Study the drawing (mm; zero at the part's minimum x, y, z) and answer. A direction names the side the tool comes from. Round coordinates to 2 decimals unless told otherwise and drop trailing zeros. Loops run counter-clockwise (first coordinate to the right, second up) from the corner with the lowest first, then second, coordinate; pieces in that order, holes last. Notation, with made-up numbers: M 14.25,57.25 L 50.25,57.25 A8 ccw 50.25,70.25 Z; hole C 35.5,-14.75 d3. An arc over 180 degrees is marked long. Put each result on its own line as item: value. Start each with the question number.
(1) Section B-B, the plane x = 2.25 is taken. Determine the outline of the cut face in (y, z), then the cut area to 4 significant figures.
(2) Determine the mould class of the marked faces 6, 7 and 8 for opening direction X: released by +X, released by -X, zero draft, split by the parting line, or undercut.
(3) Which of the six approach directions +Z, -Z, +X, -X, +Y, -Y give full straight-line access (tool end or side, diameter ignored) to the marked faces 1, 2, 3, 4 and 5?
(4) Section A-A, the plane z = 6 is taken. Determine the outline of the cut face in (x, y).
(5) Section C-C, the plane z = 10.5 is taken. Determine the outline of the cut face in (x, y).
(6) Flat-ended cylindrical pins translate along their axes: P1, Ø12, axis at x = 5.5, z = 14.5, coming from the +Y side; P2, Ø7.5, axis at x = 4, z = 18.5, coming from the -Y side; P3, Ø5, axis at x = 27, y = 16.5, coming from the +Z side. Find the tip coordinate at first contact, or state that the pin passes through.
(7) Section D-D, the plane y = 22 is taken. Determine the outline of the cut face in (x, z).
(8) Straight lines are drawn through the part: line 1 (X direction, y = 11, z = 5); line 2 (X direction, y = 27, z = 31.5); line 3 (Z direction, x = 8, y = 29.5). For each, find the intervals that lie inside material, in ascending order.
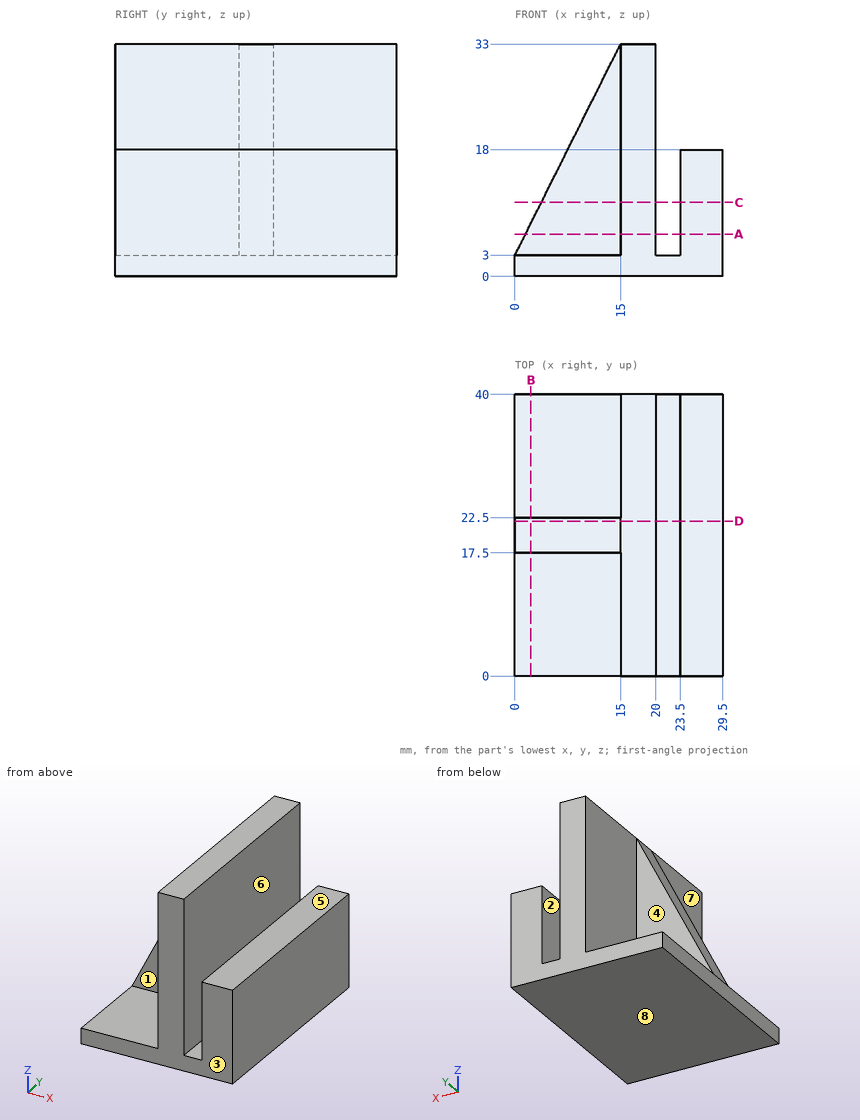
Recorded:
1. outline: M 0,0 L 40,0 L 40,3 L 22.5,3 L 22.5,7.5 L 17.5,7.5 L 17.5,3 L 0,3 Z
1. area: 142.5 mm²
2. face 6: undercut
2. face 7: released by -X
2. face 8: zero draft
3. face 1: +Z, -X, -Y
3. face 2: +Z, +Y, -Y
3. face 3: +Z, -Z, +X, -X, -Y
3. face 4: +Z, -X, +Y
3. face 5: +Z, +X, +Y, -Y
4. outline: M 1.5,17.5 L 15,17.5 L 15,0 L 20,0 L 20,40 L 15,40 L 15,22.5 L 1.5,22.5 Z; M 23.5,0 L 29.5,0 L 29.5,40 L 23.5,40 Z
5. outline: M 3.75,17.5 L 15,17.5 L 15,0 L 20,0 L 20,40 L 15,40 L 15,22.5 L 3.75,22.5 Z; M 23.5,0 L 29.5,0 L 29.5,40 L 23.5,40 Z
6. P1: stops at y = 22.5
6. P2: stops at y = 17.5
6. P3: stops at z = 18
7. outline: M 0,0 L 29.5,0 L 29.5,18 L 23.5,18 L 23.5,3 L 20,3 L 20,33 L 15,33 L 0,3 Z
8. line 1: x = 15 to 20, 23.5 to 29.5
8. line 2: x = 15 to 20
8. line 3: z = 0 to 3
